The drawing under review shows one solid part. Ordinate dimensions are in mm from its lowest x, y, z. A direction names the side the tool comes from. Coordinates: 2 decimals unless noted, no trailing zeros. Write each loop counter-clockwise with the first axis right and the second up, starting at its lowest first coordinate (ties: lowest second). Pieces come first, ordered by that corner, then holes. Notation, with made-up numbers: (-18, 31) -> (35, 31) arc R19 cw to (35, 43) -> close; hole circle Ø1 at (87, 27.25). An arc over 180 degrees is marked (long way). One line per question, with ' | ' between items. Start each with the question number.
Q1. Add section C-C on x = 27.5. State the section outline as (y, z) points.
Q2. Add section B-B on y = 27.5. State the section outline as (x, z) points, and give its area (3 significant figures).
Q3. Add section D-D on z = 3.6. State the section outline as (x, y) points (3 decimals).
Q4. For P1, Ø2.5, axis at x = 39, z = 3, coming from the +Y side; P2, Ø1.5, axis at x = 1.5, z = 3, coming from the +Y side; P3, Ø2.5, axis at y = 15.5, z = 2.5, coming from the -X side; P4, Ø1.5, axis at x = 22.42, y = 36.29, coming from the -Z side, all flat-tipped, find the tip position at first contact; note any pin that passes through.
Q5. For the marked faces 1, 2, 3, 4 and 5, list the 3-axis set-ups (+Z, -Z, +X, -X, +Y, -Y) from which the entire face can be reached by the end or side of a thin tool; tool diameter is ignored.
Q6. Add section A-A on x = 17.35. State the section outline as (y, z) points, and give its area (4 significant figures).
Q7. Draft analysis for pull direction X (two halves, no side actions). For the marked faces 6, 7, 8 and 9, state which applies: pulls with the +X half, pulls with the -X half, needs draft (parallel to the pull), parting line crosses it, or undercut.
Q8. Wall thickness on probe 1 along X at (y, z) = (42, 2.6); probe 2 along Y at (x, z) = (30, 0.85): over which ranges is each line inside the solid? List them lowest first.
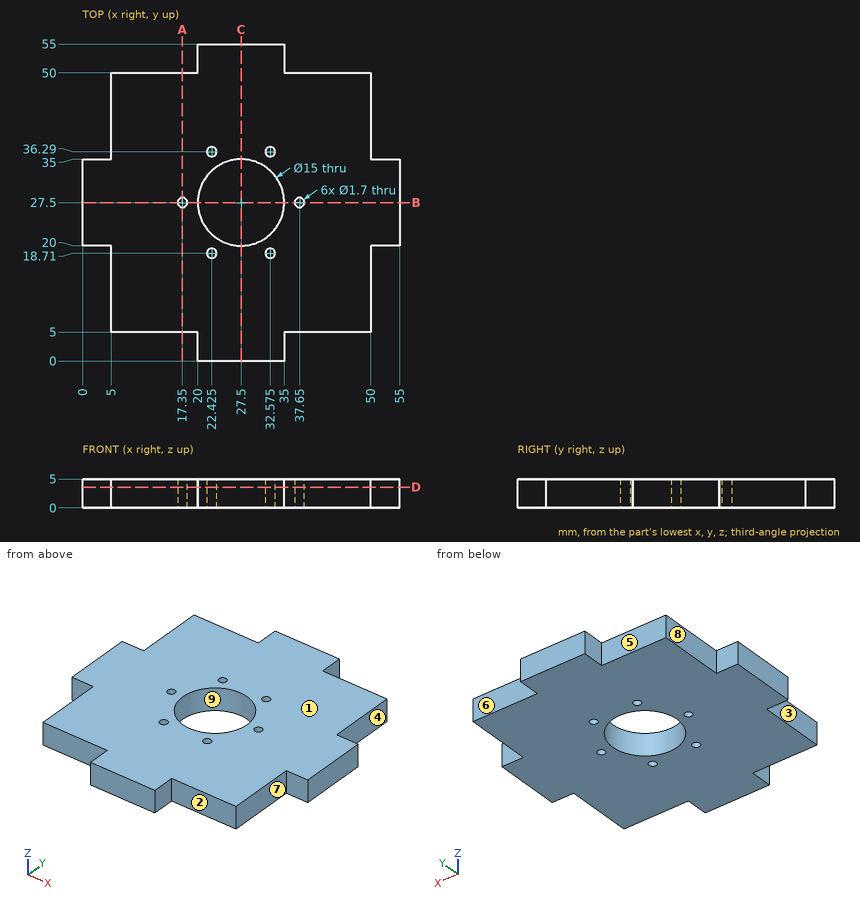
Output values:
1) outline: (0, 0) -> (20, 0) -> (20, 5) -> (0, 5) -> close; (35, 0) -> (55, 0) -> (55, 5) -> (35, 5) -> close
2) outline: (0, 0) -> (16.5, 0) -> (16.5, 5) -> (0, 5) -> close; (18.2, 0) -> (20, 0) -> (20, 5) -> (18.2, 5) -> close; (35, 0) -> (36.8, 0) -> (36.8, 5) -> (35, 5) -> close; (38.5, 0) -> (55, 0) -> (55, 5) -> (38.5, 5) -> close | area: 183 mm2
3) outline: (0, 20) -> (5, 20) -> (5, 5) -> (20, 5) -> (20, 0) -> (35, 0) -> (35, 5) -> (50, 5) -> (50, 20) -> (55, 20) -> (55, 35) -> (50, 35) -> (50, 50) -> (35, 50) -> (35, 55) -> (20, 55) -> (20, 50) -> (5, 50) -> (5, 35) -> (0, 35) -> close; hole circle Ø1.7 at (17.35, 27.5); hole circle Ø15 at (27.5, 27.5); hole circle Ø1.7 at (22.425, 18.71); hole circle Ø1.7 at (22.425, 36.29); hole circle Ø1.7 at (32.575, 18.71); hole circle Ø1.7 at (32.575, 36.29); hole circle Ø1.7 at (37.65, 27.5)
4) P1: stops at y = 50 | P2: stops at y = 35 | P3: stops at x = 5 | P4: passes through
5) face 1: +Z, +X, -X, +Y, -Y | face 2: +Z, -Z, +X, -Y | face 3: +Z, -Z, -X, -Y | face 4: +Z, -Z, +X, +Y | face 5: +Z, -Z, -X, +Y
6) outline: (5, 0) -> (26.65, 0) -> (26.65, 5) -> (5, 5) -> close; (28.35, 0) -> (50, 0) -> (50, 5) -> (28.35, 5) -> close | area: 216.5 mm2
7) face 6: needs draft | face 7: pulls with the +X half | face 8: pulls with the -X half | face 9: undercut
8) probe 1: x = 5 to 50 | probe 2: y = 0 to 20.43, 34.57 to 55
